Build history of the part. All positions in model axes, mm. Face numbers are marked on the shaded views. A direction names the side the tool comes from. Give positions to 0.01 mm unless a question says otherwise; leave off trailing zeros. Loops run counter-clockwise (first coordinate to the right, second up) from the corner with the lowest first, then second, coordinate; pieces in that order, holes last. Notation, with made-up numbers: (-16, 15) - (-3, 15) arc R22 ccw to (-3, 54) - close; hole circle Ø9 at (82, 67). An arc over 180 degrees is marked (long way). Return JSON: item names as keys, results as strings. Group by question number.
1) 3-axis set-ups, long thin cutter, end or side, ignore diameter. For the marked faces 4 and 5: which of +Z, -Z, +X, -X, +Y, -Y reach the whole face in a straight line?
2) Drop flat-ended pins along their axis: pin 1 (3 mm diameter, centred on x = 14.5, z = -6, fed in from -Y); pin 2 (1.5 mm diameter, centred on y = -14.5, z = -5.5, fed in from +X); pin 3 (2 mm diameter, centred on x = 17, y = -12, fed in from +Z); pin 4 (1 mm diameter, centred on y = 20.5, z = -4.5, fed in from +X). Give the stop position or say it passes through.
3) Slice it at A-A (y = 0). List the corners of the cut face in (x, z).
4) Drill centre lines: probe 1 along X at (y, z) = (0, -2.6); probe 2 along Y at (x, z) = (7.5, -3.5); probe 3 along X at (y, z) = (-14.5, -6). Where is each one in solid material? Low to high. Write a range as from..to.
5) Slice it at D-D (y = 22.5). List the corners of the cut face in (x, z).
6) Slice it at C-C (z = -4.75). List the corners of the cut face in (x, y), and give its area (3 significant figures).
7) Mould opens along Z. For the marked faces 1, 2 and 3 say: released by +Z, released by -Z, zero draft, split by the parting line, or undercut.
```python
from build123d import *


with BuildPart() as part:
    # Sketch1 → Revolve1 (revolve)
    with BuildSketch(Plane(origin=(0, 0, 0), x_dir=(0, 0, -1), z_dir=(1, 0, 0))):
        Polygon((8, 26), (0, 26), (0, 18.157077096), (1.289905359, 18.157077096), (0.646560904, 16.300067014), (1.512702621, 16), (2.240654576, 18.101229145), (3.267168994, 18.101229145), (6.501757282, 16), (7.719119992, 18.162900408), (7.719119992, 19.256131168), (1.470175501, 19.256131168), (1.470175501, 24.294482866), (8, 24.294482866), align=None)
    revolve(axis=Axis((0, 0, 0), (0, 0, -1)))


solid = part.part
```
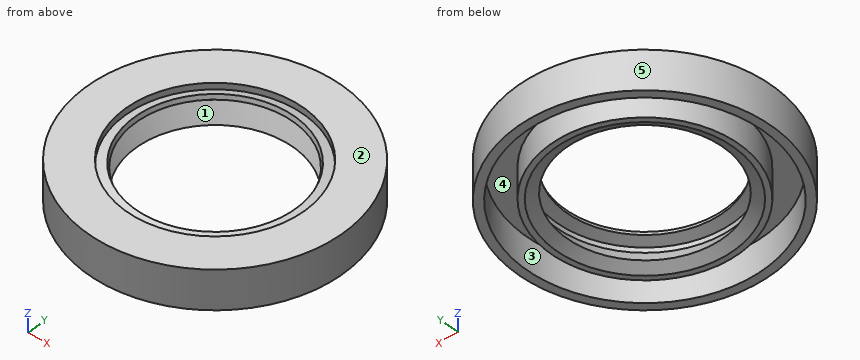
Results:
{
 "1": {"face 4": "-Z", "face 5": "+Z, -Z"},
 "2": {"pin 1": "y = -22.52", "pin 2": "x = 22.07", "pin 3": "z = 0", "pin 4": "x = 16.61"},
 "3": {"outline": "(-26, -8) - (-24.29, -8) - (-24.29, -1.47) - (-19.26, -1.47) - (-19.26, -7.72) - (-18.16, -7.72) - (-16, -6.5) - (-18.1, -3.27) - (-18.1, -2.24) - (-16, -1.51) - (-16.3, -0.65) - (-18.16, -1.29) - (-18.16, 0) - (-26, 0) - close; (16, -6.5) - (18.16, -7.72) - (19.26, -7.72) - (19.26, -1.47) - (24.29, -1.47) - (24.29, -8) - (26, -8) - (26, 0) - (18.16, 0) - (18.16, -1.29) - (16.3, -0.65) - (16, -1.51) - (18.1, -2.24) - (18.1, -3.27) - close"},
 "4": {"probe 1": "-26..-24.29, -19.26..-18.1, 18.1..19.26, 24.29..26", "probe 2": "-24.89..-23.11, -17.74..-16.31, 16.31..17.74, 23.11..24.89", "probe 3": "-21.58..-19.49, -12.67..-7.5, 7.5..12.67, 19.49..21.58"},
 "5": {"outline": "(-13.03, -8) - (-9.16, -8) - (-9.16, -1.47) - (9.16, -1.47) - (9.16, -8) - (13.03, -8) - (13.03, 0) - (-13.03, 0) - close"},
 "6": {"outline": "circle Ø52 at (0, 0); circle Ø38.51 at (0, 0); hole circle Ø48.59 at (0, 0); hole circle Ø34.28 at (0, 0)", "area": "512 mm2"},
 "7": {"face 1": "undercut", "face 2": "released by +Z", "face 3": "zero draft"}
}
